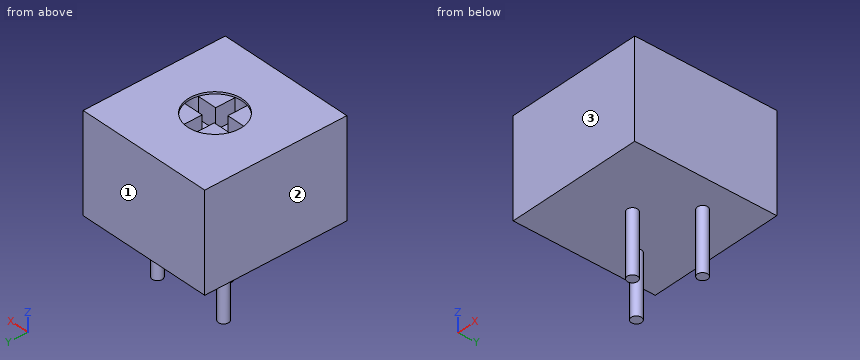
```python
from build123d import *

# Parameters (mm, degrees)
SKETCH_1_W          = 6.6
SKETCH_1_H          = 6.9
EXTRUDE_1_DEPTH     = 4.7
SKETCH_2_R          = 1.32
CUT_EXTRUDE_1_DEPTH = 0.1
CUT_EXTRUDE_2_DEPTH = 1
SKETCH_4_R          = 0.25
EXTRUDE_2_DEPTH     = 3


with BuildPart() as part:
    # Эскиз1 → Бобышка-Вытянуть1 (new body)
    with BuildSketch(Plane.XY):
        Rectangle(SKETCH_1_W, SKETCH_1_H)
    extrude(amount=EXTRUDE_1_DEPTH)

    # Эскиз2 → Вырез-Вытянуть1 (cut)
    with BuildSketch(Plane.XY.offset(4.7)):
        Circle(SKETCH_2_R)
    extrude(amount=-CUT_EXTRUDE_1_DEPTH, mode=Mode.SUBTRACT)

    # Эскиз3 → Вырез-Вытянуть2 (cut)
    with BuildSketch(Plane.XY.offset(4.6)):
        with BuildLine():
            Line((-0.33, 1.278084504), (-0.33, 0.33))
            Line((-0.33, 0.33), (-1.278084504, 0.33))
            ThreePointArc((-1.278084504, 0.33), (-1.32, 0), (-1.278084504, -0.33))
            Line((-1.278084504, -0.33), (-0.33, -0.33))
            Line((-0.33, -0.33), (-0.33, -1.278084504))
            ThreePointArc((-0.33, -1.278084504), (0, -1.32), (0.33, -1.278084504))
            Line((0.33, -1.278084504), (0.33, -0.33))
            Line((0.33, -0.33), (1.278084504, -0.33))
            ThreePointArc((1.278084504, -0.33), (1.32, 0), (1.278084504, 0.33))
            Line((1.278084504, 0.33), (0.33, 0.33))
            Line((0.33, 0.33), (0.33, 1.278084504))
            ThreePointArc((0.33, 1.278084504), (0, 1.32), (-0.33, 1.278084504))
        make_face()
    extrude(amount=-CUT_EXTRUDE_2_DEPTH, mode=Mode.SUBTRACT)

    # Эскиз4 → Бобышка-Вытянуть2 (add)
    with BuildSketch(Plane.XY):
        with Locations((1.79605, 1.19)):
            Circle(SKETCH_4_R)
        with Locations((-1.79605, 1.19)):
            Circle(SKETCH_4_R)
        with Locations((0, -0.61)):
            Circle(SKETCH_4_R)
    extrude(amount=-EXTRUDE_2_DEPTH)


solid = part.part
```
Model file for the job. Use its own axes, mm. Face numbers are marked on the shaded views. Give positions to 0.01 mm unless a question says otherwise; leave off trailing zeros. Write each loop counter-clockwise with the first axis right and the second up, starting at its lowest first coordinate (ties: lowest second). Pieces come first, ordered by that corner, then holes. Notation, with made-up numbers: (60, 2) - (112, 2) arc R16 ccw to (112, 25) - close; hole circle Ø10 at (47.25, 45.25). An arc over 180 degrees is marked (long way). One line per question, with ' | ' between items. Start each with the question number.
(1) Slice it at B-B on x = 0. Write the cut outline in (y, z), plus the area to 3 significant figures.
(2) Pin check, flat tip, straight feed: P1, Ø1.3, axis at x = 0, y = 0, coming from the +Z side. Stop position of the tip, or through.
(3) Two-plate mould, pull along Y, no slides. Class the marked faces 1, 2 and 3: +Y half, -Y half, draft (parallel to the pull), parting line (faces both ways), or undercut.
(4) Wall check: line 1 along Y through (x, z) = (0, 4.25); line 2 along X through (y, z) = (0, 4.1); line 3 along Y through (x, z) = (0.75, 4). Give the ranges that are in metal, low to high. Write a range as from..to.
(5) Slice it at A-A on y = 0. Write the cut outline in (x, z).
(6) Slice it at C-C on x = 2.25. Write the cut outline in (y, z).
(7) Slice it at D-D on y = 2.5. Write the cut outline in (x, z), plus the area to 3 significant figures.
Results below:
1) outline: (-3.45, 0) - (-0.86, 0) - (-0.86, -3) - (-0.36, -3) - (-0.36, 0) - (3.45, 0) - (3.45, 4.7) - (1.32, 4.7) - (1.32, 3.6) - (-1.32, 3.6) - (-1.32, 4.7) - (-3.45, 4.7) - close | area: 31.0 mm^2
2) P1: z = 4.6
3) face 1: +Y half | face 2: draft | face 3: -Y half
4) line 1: -3.45..-1.32, 1.32..3.45 | line 2: -3.3..-1.32, 1.32..3.3 | line 3: -3.45..-0.33, 0.33..3.45
5) outline: (-3.3, 0) - (3.3, 0) - (3.3, 4.7) - (1.32, 4.7) - (1.32, 3.6) - (-1.32, 3.6) - (-1.32, 4.7) - (-3.3, 4.7) - close
6) outline: (-3.45, 0) - (3.45, 0) - (3.45, 4.7) - (-3.45, 4.7) - close
7) outline: (-3.3, 0) - (3.3, 0) - (3.3, 4.7) - (-3.3, 4.7) - close | area: 31.0 mm^2
